Drawing for the job (mm, zero at the part's lowest x, y, z). Round coordinates to 2 decimals unless told otherwise and drop trailing zeros. Order: outer loops, then holes, each group sorted by start corner. A loop starts at its lowest first (then second) coordinate and runs counter-clockwise, first axis right, second up. Notation, with made-up numbers: M 64,39.25 L 118,39.25 A31 ccw 118,66.25 Z; hole C 39.5,22.25 d3. An arc over 180 degrees is marked long. Answer as CSV lines item,"result". Start each with the question number.
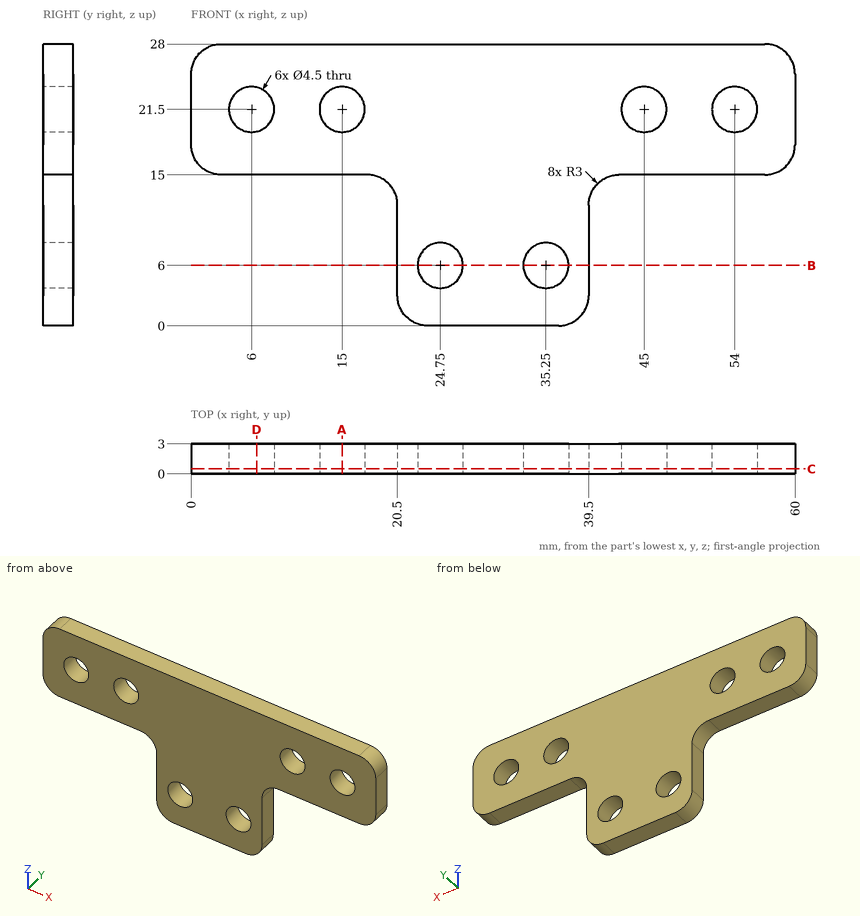
Q1. Drop flat-ended pins along their axis: P1, Ø0.9, axis at y = 2, z = 9, coming from the -X side; P2, Ø2.5, axis at x = 54, z = 21.5, coming from the +Y side; P3, Ø0.9, axis at x = 11, y = 1.5, coming from the -Z side; P4, Ø0.9, axis at y = 1, z = 9.5, coming from the +X side. Give the stop position or say it passes through.
Q2. Band-saw the part on D-D, the plane x = 6.5. Write the cut outline in (y, z), then the cut area to 3 significant figures.
Q3. Probe line 1 along X through (y, z) = (1.2, 21.5); line 2 along X through (y, z) = (2.35, 6); line 3 along Z through (x, y) = (6, 1). List the from-to ranges inside material, lowest first. Write a range as from..to.
Q4. Band-saw the part on B-B, the plane z = 6. Write the cut outline in (x, y), then the cut area to 3 significant figures.
Q5. Band-saw the part on A-A, the plane x = 15. Write the cut outline in (y, z).
Q6. Band-saw the part on C-C, the plane y = 0.5. Write the cut outline in (x, z), then the cut area to 3 significant figures.
Answer:
1,P1,"stops at x = 20.5"
1,P2,"passes through"
1,P3,"stops at z = 15"
1,P4,"stops at x = 39.5"
2,outline,"M 0,15 L 3,15 L 3,19.31 L 0,19.31 Z; M 0,23.69 L 3,23.69 L 3,28 L 0,28 Z"
2,area,"25.8 mm^2"
3,line 1,"x = 0..3.75, 8.25..12.75, 17.25..42.75, 47.25..51.75, 56.25..60"
3,line 2,"x = 20.5..22.5, 27..33, 37.5..39.5"
3,line 3,"z = 15..19.25, 23.75..28"
4,outline,"M 20.5,0 L 22.5,0 L 22.5,3 L 20.5,3 Z; M 27,0 L 33,0 L 33,3 L 27,3 Z; M 37.5,0 L 39.5,0 L 39.5,3 L 37.5,3 Z"
4,area,"30.0 mm^2"
5,outline,"M 0,15 L 3,15 L 3,19.25 L 0,19.25 Z; M 0,23.75 L 3,23.75 L 3,28 L 0,28 Z"
6,outline,"M 0,18 A3 ccw 3,15 L 17.5,15 A3 cw 20.5,12 L 20.5,3 A3 ccw 23.5,0 L 36.5,0 A3 ccw 39.5,3 L 39.5,12 A3 cw 42.5,15 L 57,15 A3 ccw 60,18 L 60,25 A3 ccw 57,28 L 3,28 A3 ccw 0,25 Z; hole C 6,21.5 d4.5; hole C 15,21.5 d4.5; hole C 24.75,6 d4.5; hole C 35.25,6 d4.5; hole C 45,21.5 d4.5; hole C 54,21.5 d4.5"
6,area,"962 mm^2"
